For this review, take the finished solid that the model builds, in its own axes (mm). Face numbers are marked on the shaded views. A direction names the side the tool comes from. Give positions to 0.01 mm unless a question says otherwise; leave off trailing zeros. Order: outer loops, then holes, each group sorted by start corner. A loop starts at its lowest first (then second) coordinate and runs counter-clockwise, first axis right, second up. Notation, with made-up numbers: (62.25, 27.5) - (112.25, 27.5) arc R14 cw to (112.25, 53.5) - close; hole circle Ø7 at (-1.5, 68.25). An arc over 180 degrees is marked (long way). Use a Markdown table: item, result. Add a question column.
1) We need section D-D on z = 680. Write out the cut boundary in (x, y), then the cut area to 3 significant figures.
2) Wall thickness on L1, parallel to Y at x = 78, z = 705.5; L2, parallel to Z at x = 107.5, y = -438; L3, parallel to Y at x = 59.5, z = 431.5: over which ranges is each line inside the solid? List them lowest first.
3) We need section B-B on x = 12. Write out the cut boundary in (y, z), then the cut area to 3 significant figures.
4) We need section C-C on y = 325. Write out the cut boundary in (x, z), then the cut area to 4 significant figures.
5) Machinability: for the marked faces 1, 2 and 3, which of the approach directions +Z, -Z, +X, -X, +Y, -Y give a long, thin tool a straight path to every point of the face, cutting with its end or side? Answer none if there is none.
6) Clearance check with flat-ended pins moving along their axes: P1, Ø10, axis at x = 74.5, y = 452.5, coming from the -Z side; P2, Ø5, axis at x = 66, z = 630.5, coming from the -Y side. State where each tip first meets the part, or that it passes through.
7) We need section A-A on z = 582.5. Write out the cut boundary in (x, y), then the cut area to 3 significant figures.
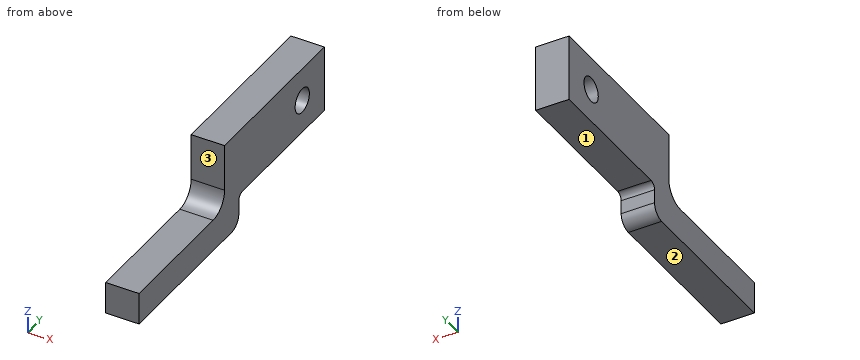
```python
from build123d import *

# Parameters (mm, degrees)
BOSS_EXTRUDE1_DEPTH = 135
SKETCH2_W           = 135
SKETCH2_H           = 270
BOSS_EXTRUDE2_DEPTH = 300
SKETCH3_R           = 50
CUT_EXTRUDE1_DEPTH  = 1070.285321259


with BuildPart() as part:
    # Sketch1 → Boss-Extrude1 (new body)
    with BuildSketch(Plane(origin=(0, 0, 0), x_dir=(0, 0, -1), z_dir=(1, 0, 0))):
        with BuildLine():
            Line((-465.792131575, 464.039290463), (-465.792131575, 189.039290463))
            ThreePointArc((-465.792131575, 189.039290463), (-458.469801105, 171.361620934), (-440.792131575, 164.039290463))
            Line((-440.792131575, 164.039290463), (-385.792131575, 164.039290463))
            ThreePointArc((-385.792131575, 164.039290463), (-350.436792516, 149.394629523), (-335.792131575, 114.039290463))
            Line((-335.792131575, 114.039290463), (-335.792131575, -535.960709537))
            Line((-335.792131575, -535.960709537), (-465.792131575, -535.960709537))
            Line((-465.792131575, -535.960709537), (-465.792131575, -15.960709537))
            ThreePointArc((-465.792131575, -15.960709537), (-489.22358908, 40.607832958), (-545.792131575, 64.039290463))
            Line((-545.792131575, 64.039290463), (-735.792131575, 64.039290463))
            Line((-735.792131575, 64.039290463), (-735.792131575, 464.039290463))
            Line((-735.792131575, 464.039290463), (-465.792131575, 464.039290463))
        make_face()
    extrude(amount=BOSS_EXTRUDE1_DEPTH)

    # Sketch2 → Boss-Extrude2 (add)
    with BuildSketch(Plane(origin=(0, 464.039290463, 0), x_dir=(1, 0, 0), z_dir=(0, 1, 0))):
        with Locations((67.5, -600.792131575)):
            Rectangle(SKETCH2_W, SKETCH2_H)
    extrude(amount=BOSS_EXTRUDE2_DEPTH)

    # Sketch3 → Cut-Extrude1 (cut, through all)
    with BuildSketch(Plane(origin=(135, 0, 0), x_dir=(0, 0, -1), z_dir=(1, 0, 0))):
        with Locations((-600.792131575, 609.039290463)):
            Circle(SKETCH3_R)
    extrude(amount=-CUT_EXTRUDE1_DEPTH, mode=Mode.SUBTRACT)


solid = part.part
```
Checked values:
| question | item | result |
|---|---|---|
| 1 | outline | (0, 64.04) - (135, 64.04) - (135, 764.04) - (0, 764.04) - close |
| 1 | area | 94,500 mm² |
| 2 | L1 | 64.04 to 764.04 |
| 2 | L2 | 335.79 to 465.79 |
| 2 | L3 | -535.96 to 164.04 |
| 3 | outline | (-535.96, 335.79) - (114.04, 335.79) arc R50 ccw to (164.04, 385.79) - (164.04, 440.79) arc R25 cw to (189.04, 465.79) - (764.04, 465.79) - (764.04, 735.79) - (64.04, 735.79) - (64.04, 545.79) arc R80 cw to (-15.96, 465.79) - (-535.96, 465.79) - close; hole circle Ø100 at (609.04, 600.79) |
| 3 | area | 273,000 mm² |
| 4 | outline | (0, 465.79) - (135, 465.79) - (135, 735.79) - (0, 735.79) - close |
| 4 | area | 36,450 mm² |
| 5 | face 1 | -Z, +X, -X, +Y |
| 5 | face 2 | -Z, +X, -X, +Y, -Y |
| 5 | face 3 | +Z, +X, -X, -Y |
| 6 | P1 | z = 465.79 |
| 6 | P2 | y = 64.04 |
| 7 | outline | (0, 64.04) - (135, 64.04) - (135, 562.51) - (0, 562.51) - close; (0, 655.57) - (135, 655.57) - (135, 764.04) - (0, 764.04) - close |
| 7 | area | 81,900 mm² |
